Input: part model. Units: mm. Frame: model coordinates. Coordinates: 2 decimals unless noted, no trailing zeros. Write each loop counter-clockwise with the first axis right and the second up, starting at its lowest first coordinate (ties: lowest second). Pieces come first, ordered by that corner, then holes. Notation, with made-up numbers: (-20, 61) - (-12, 61) arc R23 cw to (-12, 71) - close; hole circle Ø10 at (10.25, 78.5). An arc over 180 degrees is marked (long way). Put each result on its own line as item: value. Start each with the question number.
1. Cut plane A-A, the plane z = 1.4. Return loops of the section in (x, y).
2. Pin query (flat end, axial travel): pin 1 (1 mm diameter, centred on y = 58.5, z = 1, fed in from -X); pin 2 (4 mm diameter, centred on x = -208.16, y = 56.68, fed in from -Z); pin 3 (1 mm diameter, centred on y = 58.5, z = 1.5, fed in from +X). Return the tip coordinate at first contact, or that it passes through.
3. Pull-direction query (X, two-part tool) for faces 1 (the cylindrical face through (1.84, 56.79, 1.48)), 2 (the flat face through (-115, 57, 3)), 3 (the cylindrical face through (-3.615, 58.726, 1.479)); classes: released by +X, released by -X, zero draft, split by the parting line, or undercut.
4. Line query: line 1 (X direction, y = 59, z = 0.4); line 2 (X direction, y = 54.75, z = 0.95); line 3 (X direction, y = 55.25, z = 2). Output: solid intervals per line, ascending.
Autodesk Inventor part; units mm, degrees
ref_plane "YZ Plane" through (0, 0, 0) normal (1, 0, 0) x (0, 1, 0)
ref_plane "XZ Plane" through (0, 0, 0) normal (0, 1, 0) x (-1, 0, 0)
ref_plane "XY Plane" through (0, 0, 0) normal (0, 0, 1) x (1, 0, 0)
sketch "草圖1" plane through (0, 0, 0) normal (0, 0, 1) x (1, 0, 0)
  line L0 (-223.1596, 56.676) -> (-3.1596, 56.676) construction
  line L1 (-223.1596, 51.676) -> (-3.1596, 51.676)
  line L2 (-3.1596, 61.676) -> (-223.1596, 61.676)
  arc A0 (-223.1596, 61.676) -> (-223.1596, 51.676) centre (-223.1596, 56.676) ccw
  arc A1 (-3.1596, 51.676) -> (-3.1596, 61.676) centre (-3.1596, 56.676) ccw
  circle A2 centre (-223.1596, 56.676) radius 2.1
  circle A3 centre (-3.1596, 56.676) radius 2.1
  circle A4 centre (-208.1596, 56.676) radius 2.1
  circle A5 centre (-53.1596, 56.676) radius 3.5
  line L3 (-223.1596, 61.676) -> (-222.1596, 61.676)
  line L4 (-222.1596, 61.676) -> (-222.1596, 58.5227)
  line L5 (-222.1596, 58.5227) -> (-223.1596, 58.5227)
  line L6 (-223.1596, 58.5227) -> (-223.1596, 61.676)
  point P0 (0, 0)
  point P1 (-113.1596, 56.676)
  point P2 (-223.1596, 58.776)
  dimension "d2" = 4.2
  dimension "d0" = 220
  dimension "d1" = 10
  dimension "d3" = 4.2
  dimension "d4" = 4.2
  dimension "d5" = 15
  dimension "d8" = 7
  dimension "d9" = 50
  dimension "d10" = 1
extrude "擠出1" add sketch "草圖1" along normal blind 3 contours A0 L6 A2 L4 L2 A1 L1
Report:
1. outline: (-223.16, 51.68) - (-3.16, 51.68) arc R5 ccw to (-3.16, 61.68) - (-222.16, 61.68) - (-222.16, 58.52) arc R2.1 cw (long way) to (-223.16, 58.78) - (-223.16, 61.68) arc R5 ccw to start; hole circle Ø4.2 at (-208.16, 56.68); hole circle Ø7 at (-53.16, 56.68); hole circle Ø4.2 at (-3.16, 56.68)
2. pin 1: stops at x = -227.98
2. pin 2: passes through
2. pin 3: stops at x = 1.66
3. face 1: released by +X
3. face 2: zero draft
3. face 3: undercut
4. line 1: x = -227.59 to -223.16, -222.16 to -55.78, -50.54 to 1.27
4. line 2: x = -227.77 to -224, -222.32 to -209, -207.32 to -56.08, -50.24 to -4, -2.32 to 1.45
4. line 3: x = -227.95 to -224.7, -221.62 to -209.7, -206.62 to -56.36, -49.96 to -4.7, -1.62 to 1.63
